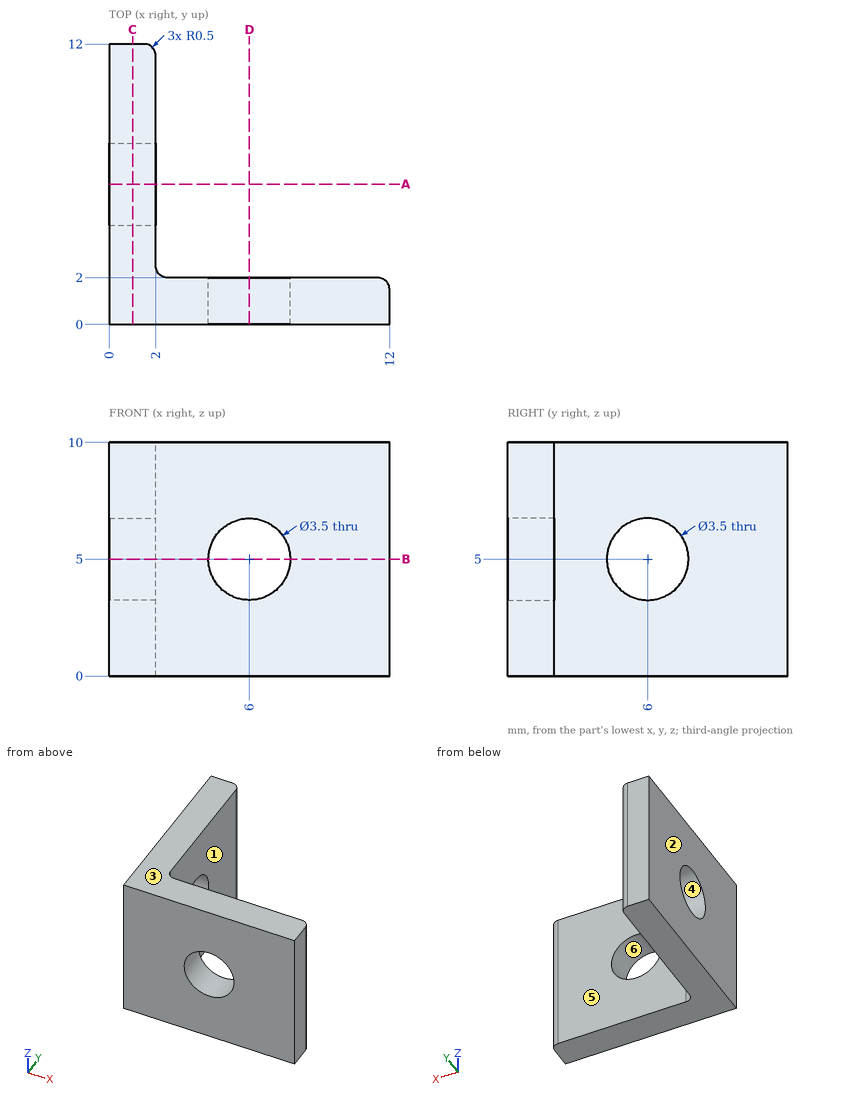
Answer from the drawing. Dimensions are ordinates in mm from the lowest x, y and z of the part. A direction names the side the tool comes from. Coordinates: 2 decimals unless noted, no trailing zeros. Order: outer loops, then holes, each group sorted by start corner. A loop starts at its lowest first (then second) coordinate and runs counter-clockwise, first axis right, second up. Notation, with made-up numbers: M 53.25,-23 L 57.25,-23 A17 cw 57.25,-12 Z; hole C 36.25,14.5 d8. An arc over 180 degrees is marked long. Put each result on its own line as item: value. Start each with the question number.
Item 1: Consider probe 1 along Y at (x, z) = (1.4, 5); probe 2 along X at (y, z) = (2.5, 3.5). Determine where each line is inside the solid, lowest interval first. Write a range as [from, to].
Item 2: The mould has two halves that part along Z. Classify the marked faces 3, 4, 5 and 6: +Z half, -Z half, draft (parallel to the pull), parting line (faces both ways), or undercut.
Item 3: For the marked faces 1 and 2, determine the directions among +Z, -Z, +X, -X, +Y, -Y from which every point of the face is accessible in a straight line to the end or side of a thin tool.
Item 4: Section C-C, the plane x = 1 is taken. Determine the outline of the cut face in (y, z).
Item 5: Section B-B, the plane z = 5 is taken. Determine the outline of the cut face in (x, y), plus the area to 3 significant figures.
Item 6: Section A-A, the plane y = 6 is taken. Determine the outline of the cut face in (x, z).
Item 7: Given pin 1 Ø4 at (y, z) = (5.5, 6.5) entering from -X; pin 2 Ø4 at (x, z) = (6, 5) entering from +Y; pin 3 Ø6 at (y, z) = (9, 2) entering from +X, each flat-ended and moving along its own axis, determine where each tip first touches the part or whether it passes through.
Computed:
1. probe 1: y = [0, 4.25], [7.75, 12]
1. probe 2: x = [0, 2]
2. face 3: +Z half
2. face 4: undercut
2. face 5: draft
2. face 6: undercut
3. face 1: +Z, -Z, +X, +Y
3. face 2: +Z, -Z, -X, +Y, -Y
4. outline: M 0,0 L 12,0 L 12,10 L 0,10 Z; hole C 6,5 d3.5
5. outline: M 0,0 L 4.25,0 L 4.25,2 L 2.5,2 A0.5 cw 2,2.5 L 2,4.25 L 0,4.25 Z; M 0,7.75 L 2,7.75 L 2,11.5 A0.5 ccw 1.5,12 L 0,12 Z; M 7.75,0 L 12,0 L 12,1.5 A0.5 ccw 11.5,2 L 7.75,2 Z
5. area: 29.9 mm2
6. outline: M 0,0 L 2,0 L 2,3.25 L 0,3.25 Z; M 0,6.75 L 2,6.75 L 2,10 L 0,10 Z
7. pin 1: stops at x = 0
7. pin 2: stops at y = 2
7. pin 3: stops at x = 2
